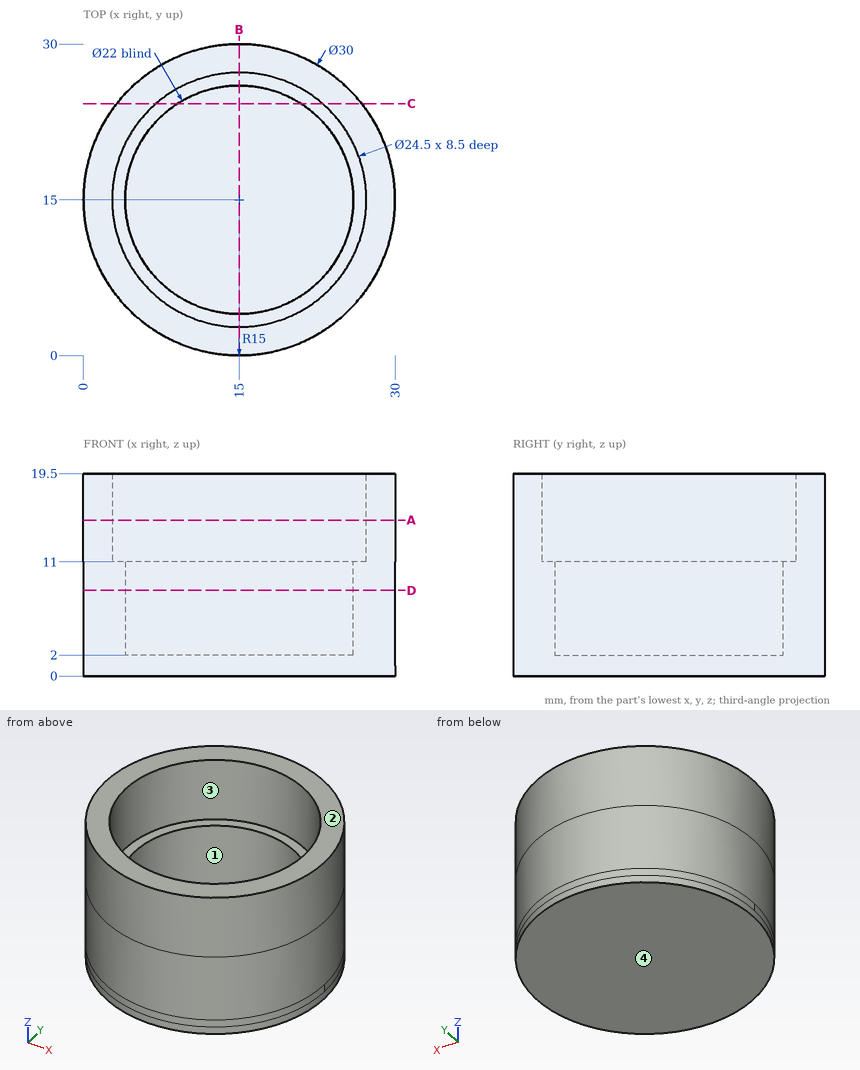
Answer from the drawing. Dimensions are ordinates in mm from the lowest x, y and z of the part. A direction names the side the tool comes from. Coordinates: 2 decimals unless noted, no trailing zeros. Order: outer loops, then holes, each group sorted by start corner. A loop starts at its lowest first (then second) coordinate and runs counter-clockwise, first axis right, second up. Notation, with made-up numbers: M 75.5,73.25 L 95.5,73.25 A14 cw 95.5,86.25 Z; hole C -6.75,69.5 d11. An arc over 180 degrees is marked long. Put each result on its own line as item: value. Start each with the question number.
Item 1: Section A-A, the plane z = 15 is taken. Determine the outline of the cut face in (x, y), plus the area to 3 significant figures.
Item 2: Given pin 1 Ø3 at (x, z) = (25.5, 5.5) entering from -Y; pin 2 Ø13 at (x, y) = (15, 15) entering from +Z; pin 3 Ø6 at (x, y) = (17, 5.5) entering from +Z; pin 4 Ø3 at (y, z) = (7, 3) entering from -X, each flat-ended and moving along its own axis, determine where each tip first touches the part or whether it passes through.
Item 3: Section B-B, the plane x = 15 is taken. Determine the outline of the cut face in (y, z), plus the area to 3 significant figures.
Item 4: For the marked faces 3 and 4, determine the directions among +Z, -Z, +X, -X, +Y, -Y from which every point of the face is accessible in a straight line to the end or side of a thin tool.
Item 5: Section C-C, the plane y = 24.25 is taken. Determine the outline of the cut face in (x, z), plus the area to 3 significant figures.
Item 6: The mould has two halves that part along Y. Classify the marked faces 1 and 2: +Y half, -Y half, draft (parallel to the pull), parting line (faces both ways), or undercut.
Item 7: Section D-D, the plane z = 8.25 is taken. Determine the outline of the cut face in (x, y), plus the area to 3 significant figures.
Item 8: Consider probe 1 along X at (y, z) = (15, 7); probe 2 along Y at (x, z) = (15, 17.75). Determine where each line is inside the solid, lowest interval first. Write a range as [from, to].
Computed:
1. outline: C 15,15 d30; hole C 15,15 d24.5
1. area: 235 mm2
2. pin 1: stops at y = 3
2. pin 2: stops at z = 2
2. pin 3: stops at z = 19.5
2. pin 4: stops at x = 1.48
3. outline: M 0,0 L 30,0 L 30,19.5 L 27.25,19.5 L 27.25,11 L 26,11 L 26,2 L 4,2 L 4,11 L 2.75,11 L 2.75,19.5 L 0,19.5 Z
3. area: 179 mm2
4. face 3: +Z
4. face 4: -Z, +X, -X, +Y, -Y
5. outline: M 3.19,0 L 26.81,0 L 26.81,19.5 L 23.03,19.5 L 23.03,11 L 20.95,11 L 20.95,2 L 9.05,2 L 9.05,11 L 6.97,11 L 6.97,19.5 L 3.19,19.5 Z
5. area: 217 mm2
6. face 1: undercut
6. face 2: draft
7. outline: C 15,15 d30; hole C 15,15 d22
7. area: 327 mm2
8. probe 1: x = [0, 4], [26, 30]
8. probe 2: y = [0, 2.75], [27.25, 30]
